```python
from build123d import *

# Parameters (mm, degrees)
F0_W      = 150
F0_H      = 80
F1_DEPTH  = 40
F2_W      = 147
F2_H      = 77
F3_DEPTH  = 38.5
F4_R      = 2.5
F5_DEPTH  = 5
F6_R      = 1.5
F7_R      = 1.5
F8_R      = 1.5
F9_R      = 1.5
F10_DEPTH = 5
F11_R     = 2.5
F12_DEPTH = 3
F13_W     = 6
F13_H     = 6
F14_DEPTH = 38.5
F15_R     = 1.5
F16_DEPTH = 35
F17_R     = 2.99999


# Not quite as in the source:
# - a fillet or chamfer is up to 0.001 mm smaller than in the source, because OpenCascade refuses the exact size


with BuildPart() as f1:
    # F0 (on Front) → F1 (new body)
    with BuildSketch(Plane.XZ):
        Rectangle(F0_W, F0_H)
    extrude(amount=F1_DEPTH)

    # F2 (on face) → F3 (cut)
    with BuildSketch(Plane.XZ.offset(40)):
        Rectangle(F2_W, F2_H)
    extrude(amount=-F3_DEPTH, mode=Mode.SUBTRACT)

    # F4 (on face) → F5 (join)
    with BuildSketch(Plane.XZ.offset(1.5)):
        with Locations((-25.5, 31)):
            Circle(F4_R)
        with Locations((-25.5, -31)):
            Circle(F4_R)
        with Locations((25.5, 31)):
            Circle(F4_R)
        with Locations((25.5, -31)):
            Circle(F4_R)
    extrude(amount=F5_DEPTH)

    # F6 (on face) + F7 (on face) + F8 (on face) + F9 (on face) → F10 (join)
    with BuildSketch(Plane.XZ.offset(6.5)):
        with Locations((-25.5, 31)):
            Circle(F6_R)
    with BuildSketch(Plane.XZ.offset(6.5)):
        with Locations((25.5, 31)):
            Circle(F7_R)
    with BuildSketch(Plane.XZ.offset(6.5)):
        with Locations((-25.5, -31)):
            Circle(F8_R)
    with BuildSketch(Plane.XZ.offset(6.5)):
        with Locations((25.5, -31)):
            Circle(F9_R)
    extrude(amount=F10_DEPTH)

    # F11 (on face) → F12 (cut)
    with BuildSketch(Plane.YZ.offset(75)):
        with Locations((-8, -30)):
            Circle(F11_R)
    extrude(amount=-F12_DEPTH, mode=Mode.SUBTRACT)

    # F13 (on face) → F14 (join)
    with BuildSketch(Plane.XZ.offset(1.5)):
        with Locations((-70.5, 0)):
            Rectangle(F13_W, F13_H)
        with Locations((70.5, 0)):
            Rectangle(F13_W, F13_H)
    extrude(amount=F14_DEPTH)

    # F15 (on face) → F16 (cut)
    with BuildSketch(Plane.XZ.offset(40)):
        with Locations((-70.5, 0)):
            Circle(F15_R)
        with Locations((70.5, 0)):
            Circle(F15_R)
    extrude(amount=-F16_DEPTH, mode=Mode.SUBTRACT)

    # F17 (radius 3 in the source; OpenCascade refuses exactly that, so slightly less here)
    f17_edges = [f1.edges().sort_by_distance(p)[0] for p in [
        (-67.5, -20.75, 3),
        (-67.5, -20.75, -3),
        (67.5, -20.75, -3),
        (67.5, -20.75, 3),
    ]]
    fillet(f17_edges, radius=F17_R)


solid = f1.part
```
Check sheet for the modelled part. Datum: model origin and axes. Units: mm. A direction names the side the tool comes from. Round coordinates to 2 decimals unless told otherwise and drop trailing zeros. Loops run counter-clockwise (first coordinate to the right, second up) from the corner with the lowest first, then second, coordinate; pieces in that order, holes last. Notation, with made-up numbers: (-0.5, 20.25) -> (9.5, 20.25) arc R23 cw to (9.5, 36.25) -> close; hole circle Ø6 at (3.25, -12). An arc over 180 degrees is marked (long way). Answer in a Markdown table with one row per item.
Q1. Sectioned sample at C-C on x = 46. Enter the section's corners in (y, z), then the cut area to 4 significant figures.
Data:
| item | result |
|---|---|
| outline | (-40, -40) -> (0, -40) -> (0, 40) -> (-40, 40) -> (-40, 38.5) -> (-1.5, 38.5) -> (-1.5, -38.5) -> (-40, -38.5) -> close |
| area | 235.5 mm^2 |
Q2. Sectioned sample at A-A on y = -8. Give the number of separate pieces and of enclosed holes in the cut face, then the cut area to 3 significant figures.
Data:
| item | result |
|---|---|
| separate pieces | 5 |
| enclosed holes | 2 |
| area | 752 mm^2 |
Q3. Set-up check for faces 1 (the face through (-1, 0, 1)), 2 (the face through (-1, -21, -38.5)): record each of +Z, -Z, +X, -X, +Y, -Y from which the full face is reachable in a straight line by a thin tool's end or side.
Data:
| item | result |
|---|---|
| face 1 | +Z, -Z, +X, -X, +Y |
| face 2 | -Y |
Q4. Thickness scan on L1, parallel to Z at x = -5.5, y = -17; L2, parallel to X at y = -11, z = 5; L3, parallel to Z at x = 74.7, y = -8. Record the ranges inside material, lowest first.
Data:
| item | result |
|---|---|
| L1 | z = -40 to -38.5, 38.5 to 40 |
| L2 | x = -75 to -73.5, 73.5 to 75 |
| L3 | z = -40 to -32.5, -27.5 to 40 |
Q5. Go/stop test with flat-tipped pins: P1, Ø0.9, axis at x = 70, z = -0.5, coming from the -Y side; P2, Ø1.5, axis at x = 26, z = 30.5, coming from the -Y side; P3, Ø1, axis at x = -38, z = -15.5, coming from the -Y side. Record where each tip stops, or that it passes through.
Data:
| item | result |
|---|---|
| P1 | stops at y = -5 |
| P2 | stops at y = -11.5 |
| P3 | stops at y = -1.5 |
Q6. Sectioned sample at D-D on z = 31. Enter the section's corners in (x, y).
Data:
| item | result |
|---|---|
| outline | (-75, -40) -> (-73.5, -40) -> (-73.5, -1.5) -> (-28, -1.5) -> (-28, -6.5) -> (-27, -6.5) -> (-27, -11.5) -> (-24, -11.5) -> (-24, -6.5) -> (-23, -6.5) -> (-23, -1.5) -> (23, -1.5) -> (23, -6.5) -> (24, -6.5) -> (24, -11.5) -> (27, -11.5) -> (27, -6.5) -> (28, -6.5) -> (28, -1.5) -> (73.5, -1.5) -> (73.5, -40) -> (75, -40) -> (75, 0) -> (-75, 0) -> close |
Q7. Release check for a two-part mould opening along Z. For faces 3 (the face through (74.26, -8.33, -27.52)), 4 (the face through (-75, -20, -1)) record: released by +Z, released by -Z, zero draft, split by the parting line, or undercut.
Data:
| item | result |
|---|---|
| face 3 | undercut |
| face 4 | zero draft |
